```python
from build123d import *

# Parameters (mm, degrees)
SKETCH_1_R      = 1.6
EXTRUDE_1_DEPTH = 3
FILLET_1_R      = 3


with BuildPart() as part:
    # 草图1 → 凸台-拉伸1 (new body)
    with BuildSketch(Plane(origin=(0, 0, 0), x_dir=(1, 0, 0), z_dir=(0, 1, 0))):
        with BuildLine():
            Line((-17, 57.5), (-17, 72.5))
            Line((-17, 72.5), (-30, 72.5))
            Line((-30, 72.5), (-30, 17.5))
            Line((-30, 17.5), (17, 17.5))
            Line((17, 17.5), (17, 30.5))
            Line((17, 30.5), (35, 30.5))
            Line((35, 30.5), (35, 52.5))
            Line((35, 52.5), (7.5, 52.5))
            Line((7.5, 52.5), (7.5, 37.5))
            ThreePointArc((7.5, 37.5), (-4.75, 25.25), (-17, 37.5))
            Line((-17, 37.5), (-17, 57.5))
        make_face()
        with Locations(Location((-23.5, 65, 0), (0, 0, 270))):
            Circle(SKETCH_1_R, mode=Mode.SUBTRACT)
        with Locations(Location((27.5, 45.5, 0), (0, 0, 270))):
            Circle(SKETCH_1_R, mode=Mode.SUBTRACT)
        with Locations(Location((27.5, 37.5, 0), (0, 0, 270))):
            Circle(SKETCH_1_R, mode=Mode.SUBTRACT)
        with Locations(Location((-22.619627786, 42.288152334, 0), (0, 0, 270))):
            Circle(SKETCH_1_R, mode=Mode.SUBTRACT)
        with Locations(Location((-15.361164072, 22.345687181, 0), (0, 0, 90))):
            Circle(SKETCH_1_R, mode=Mode.SUBTRACT)
        with Locations(Location((5.861164072, 22.345687181, 0), (0, 0, 270))):
            Circle(SKETCH_1_R, mode=Mode.SUBTRACT)
        with Locations(Location((13.119627786, 42.288152334, 0), (0, 0, 90))):
            Circle(SKETCH_1_R, mode=Mode.SUBTRACT)
    extrude(amount=EXTRUDE_1_DEPTH)

    # 圆角1
    fillet_1_edges = [part.edges().sort_by_distance(p)[0] for p in [
        (7.5, 1.5, -52.5),
        (35, 1.5, -52.5),
        (35, 1.5, -30.5),
        (17, 1.5, -30.5),
        (17, 1.5, -17.5),
        (-30, 1.5, -17.5),
        (-30, 1.5, -72.5),
        (-17, 1.5, -72.5),
    ]]
    fillet(fillet_1_edges, radius=FILLET_1_R)


solid = part.part
```
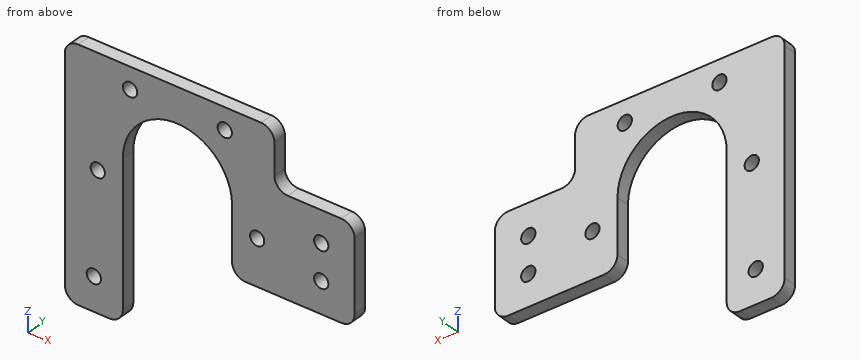
Design review of the part built by this model. Coordinates are the model's own, in mm. Give positions to 0.01 mm unless a question says otherwise; leave off trailing zeros. Order: outer loops, then holes, each group sorted by start corner. A loop starts at its lowest first (then second) coordinate and runs counter-clockwise, first axis right, second up. Notation, with made-up numbers: (-39.75, 49.25) - (-32.75, 49.25) arc R18 cw to (-32.75, 73.25) - close; hole circle Ø3 at (46, 35). An arc over 180 degrees is marked (long way). Use a Markdown table: item, result. Add a question column.
(1) Add section B-B on x = 27.5. Give the boundary of the cut face in (y, z).
(2) Wall thickness on probe 1 along X at (y, z) = (1.45, -65); probe 2 along X at (y, z) = (0.85, -38.5); probe 3 along Z at (x, y) = (28.5, 1.7): over which ranges is each line inside the solid? List them lowest first. Write a range as [from, to].
(3) Clearance check with a flat-ended pin moving along its axis: P1, Ø1, axis at y = 2.5, z = -63, coming from the +X side. State where the tip first meets the part, or that it passes through.
(4) Add section C-C on z = -22.5. Give the boundary of the cut face in (x, y).
(5) Add section A-A on z = -40. Give the boundary of the cut face in (x, y), then the cut area to 4 significant figures.
(6) Add section D-D on y = 0.8. Give the boundary of the cut face in (x, z), then the cut area to 3 significant figures.
Report:
| question | item | result |
|---|---|---|
| 1 | outline | (0, -52.5) - (3, -52.5) - (3, -47.1) - (0, -47.1) - close; (0, -43.9) - (3, -43.9) - (3, -39.1) - (0, -39.1) - close; (0, -35.9) - (3, -35.9) - (3, -30.5) - (0, -30.5) - close |
| 2 | probe 1 | x = [-30, -25.1], [-21.9, -17] |
| 2 | probe 2 | x = [-30, -17], [7.5, 26.25], [28.75, 35] |
| 2 | probe 3 | z = [-52.5, -46.75], [-44.25, -38.75], [-36.25, -30.5] |
| 3 | P1 | stops at x = -17 |
| 4 | outline | (-30, 0) - (-16.95, 0) - (-16.95, 3) - (-30, 3) - close; (-13.77, 0) - (4.27, 0) - (4.27, 3) - (-13.77, 3) - close; (7.45, 0) - (17, 0) - (17, 3) - (7.45, 3) - close |
| 5 | outline | (-30, 0) - (-17, 0) - (-17, 3) - (-30, 3) - close; (7.5, 0) - (35, 0) - (35, 3) - (7.5, 3) - close |
| 5 | area | 121.5 mm² |
| 6 | outline | (-30, -69.5) arc R3 ccw to (-27, -72.5) - (-20, -72.5) arc R3 ccw to (-17, -69.5) - (-17, -37.5) arc R12.25 cw to (7.5, -37.5) - (7.5, -49.5) arc R3 ccw to (10.5, -52.5) - (32, -52.5) arc R3 ccw to (35, -49.5) - (35, -33.5) arc R3 ccw to (32, -30.5) - (20, -30.5) arc R3 cw to (17, -27.5) - (17, -20.5) arc R3 ccw to (14, -17.5) - (-27, -17.5) arc R3 ccw to (-30, -20.5) - close; hole circle Ø3.2 at (-23.5, -65); hole circle Ø3.2 at (-22.62, -42.29); hole circle Ø3.2 at (-15.36, -22.35); hole circle Ø3.2 at (5.86, -22.35); hole circle Ø3.2 at (13.12, -42.29); hole circle Ø3.2 at (27.5, -45.5); hole circle Ø3.2 at (27.5, -37.5) |
| 6 | area | 1,630 mm² |
